Could you check a few things on this drawing? It's one solid part, dimensions in mm from its lowest x, y, z. A direction names the side the tool comes from. Give positions to 0.01 mm unless a question says otherwise; leave off trailing zeros. Loops run counter-clockwise (first coordinate to the right, second up) from the corner with the lowest first, then second, coordinate; pieces in that order, holes last. Notation, with made-up numbers: M 18,-39 L 50,-39 A19 ccw 50,-9 Z; hole C 24,-0.75 d9. An arc over 180 degrees is marked long. Answer as a JSON object with one key per item and string values.
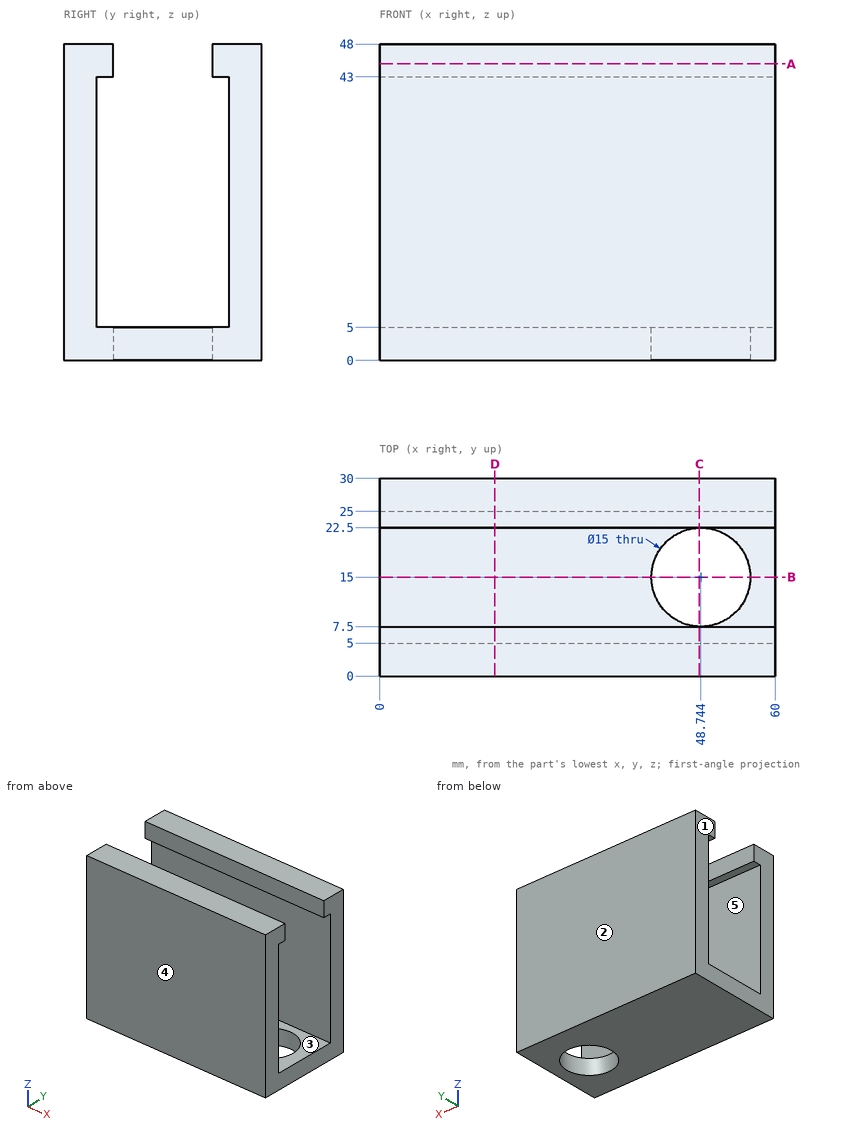
1) Suppose I cut it at C-C, the plane x = 48.5. Write out the boundary of the cut face in (y, z).
Answer list:
{"outline": "M 0,0 L 7.5,0 L 7.5,5 L 5,5 L 5,43 L 7.5,43 L 7.5,48 L 0,48 Z; M 22.5,0 L 30,0 L 30,48 L 22.5,48 L 22.5,43 L 25,43 L 25,5 L 22.5,5 Z"}
2) For the marked faces 4 and 5, which set-ups out of +Z, -Z, +X, -X, +Y, -Y let a thin tool reach every point of the face, with its end or its side?
Answer list:
{"face 4": "+Z, -Z, +X, -X, -Y", "face 5": "+X, -X"}
3) Will this pin go through, and if not, where does the flat tip stop? pin 1 Ø6 at (x, y) = (15.5, 18.5) entering from +Z.
Answer list:
{"pin 1": "z = 5"}
4) Please list where these lines run through material, in increasing order: line 1 along Z through (x, y) = (45, 6); line 2 along Y through (x, z) = (35.5, 14); line 3 along Y through (x, z) = (11, 45). Write a range as from..to.
Answer list:
{"line 1": "0..5, 43..48", "line 2": "0..5, 25..30", "line 3": "0..7.5, 22.5..30"}
5) If we mould it in two halves opening along Y, with no side actions, what happens to the marked faces 1, 2 and 3? For each: +Y half, -Y half, draft (parallel to the pull), parting line (faces both ways), or undercut.
Answer list:
{"face 1": "draft", "face 2": "+Y half", "face 3": "undercut"}
6) Suppose I cut it at D-D, the plane x = 17.5. Write out the boundary of the cut face in (y, z), and give its area (3 significant figures).
Answer list:
{"outline": "M 0,0 L 30,0 L 30,48 L 22.5,48 L 22.5,43 L 25,43 L 25,5 L 5,5 L 5,43 L 7.5,43 L 7.5,48 L 0,48 Z", "area": "605 mm^2"}
7) Suppose I cut it at A-A, the plane z = 45. Write out the boundary of the cut face in (x, y).
Answer list:
{"outline": "M 0,0 L 60,0 L 60,7.5 L 0,7.5 Z; M 0,22.5 L 60,22.5 L 60,30 L 0,30 Z"}
8) Suppose I cut it at B-B, the plane y = 15. Write out the boundary of the cut face in (x, z), and give its area (3 significant figures).
Answer list:
{"outline": "M 0,0 L 41.24,0 L 41.24,5 L 0,5 Z; M 56.24,0 L 60,0 L 60,5 L 56.24,5 Z", "area": "225 mm^2"}
